Build history of the part. All positions in model axes, mm. Round coordinates to 2 decimals unless told otherwise and drop trailing zeros. Write each loop counter-clockwise with the first axis right and the second up, starting at its lowest first coordinate (ties: lowest second). Pieces come first, ordered by that corner, then holes. Notation, with made-up numbers: (89, 60.25) -> (97, 60.25) arc R26 ccw to (97, 96.25) -> close; hole circle Ø2 at (-17, 74.25). An arc over 180 degrees is marked (long way). Answer in a Markdown table with one row per item.
```python
from build123d import *

# Parameters (mm, degrees)
BOSS_EXTRUDE1_DEPTH        = 914.4
SKETCH2_R                  = 22.225
CUT_EXTRUDE1_DEPTH         = 917.272215283
F_1_2_0_5_DIAMETER_HOLE1_D = 12.7


with BuildPart() as part:
    # Sketch1 → Boss-Extrude1 (new body)
    with BuildSketch(Plane.XY):
        with BuildLine():
            Line((41.45, -19.05), (-41.45, -19.05))
            ThreePointArc((-41.45, -19.05), (-43.571320344, -18.171320344), (-44.45, -16.05))
            Line((-44.45, -16.05), (-44.45, 16.05))
            ThreePointArc((-44.45, 16.05), (-43.571320344, 18.171320344), (-41.45, 19.05))
            Line((-41.45, 19.05), (41.45, 19.05))
            ThreePointArc((41.45, 19.05), (43.571320344, 18.171320344), (44.45, 16.05))
            Line((44.45, 16.05), (44.45, -16.05))
            ThreePointArc((44.45, -16.05), (43.571320344, -18.171320344), (41.45, -19.05))
        make_face()
    extrude(amount=BOSS_EXTRUDE1_DEPTH)

    # Sketch2 → Cut-Extrude1 (cut, through all)
    with BuildSketch(Plane(origin=(0, 19.05, 0), x_dir=(1, 0, 0), z_dir=(0, 1, 0))):
        with Locations(Location((0, -304.8, 0), (0, 0, 180))):
            Circle(SKETCH2_R)
    extrude(amount=-CUT_EXTRUDE1_DEPTH, mode=Mode.SUBTRACT)

    # 1/2 (0.5) Diameter Hole1 (through all)
    with Locations(Plane(origin=(0, 19.05, 0), x_dir=(1, 0, 0), z_dir=(0, 1, 0))):
        with Locations((-25.4, -895.35), (25.4, -895.35), (-25.4, -19.05), (25.4, -19.05)):
            Hole(F_1_2_0_5_DIAMETER_HOLE1_D / 2)


solid = part.part
```
Q1. Saw through at C-C on y = 6. Write the cut outline in (x, z) (3 decimals).
A:
| item | result |
|---|---|
| outline | (-44.45, 0) -> (44.45, 0) -> (44.45, 914.4) -> (-44.45, 914.4) -> close; hole circle Ø12.7 at (-25.4, 19.05); hole circle Ø12.7 at (-25.4, 895.35); hole circle Ø44.45 at (0, 304.8); hole circle Ø12.7 at (25.4, 19.05); hole circle Ø12.7 at (25.4, 895.35) |
Q2. Saw through at B-B on z = 304.8. Write the cut outline in (x, y) (3 decimals), plus the area to 3 significant figures.
A:
| item | result |
|---|---|
| outline | (-44.45, -16.05) arc R3 ccw to (-41.45, -19.05) -> (-22.225, -19.05) -> (-22.225, 19.05) -> (-41.45, 19.05) arc R3 ccw to (-44.45, 16.05) -> close; (22.225, -19.05) -> (41.45, -19.05) arc R3 ccw to (44.45, -16.05) -> (44.45, 16.05) arc R3 ccw to (41.45, 19.05) -> (22.225, 19.05) -> close |
| area | 1,690 mm² |
Q3. Wall check: line 1 (Z direction, x = 24, y = -5.5); line 2 (Z direction, x = 25, y = -9); line 3 (X direction, y = -1, z = 895). Give the ranges that are in metal, low to high. Write a range as [from, to].
A:
| item | result |
|---|---|
| line 1 | [0, 12.86], [25.24, 889.16], [901.54, 914.4] |
| line 2 | [0, 12.71], [25.39, 889.01], [901.69, 914.4] |
| line 3 | [-44.45, -31.74], [-19.06, 19.06], [31.74, 44.45] |
Q4. Two-plate mould, pull along X, no slides. Class faces 1 (the flat face through (44.45, 0, 451)), 2 (the cylindrical face through (4.8, 0.3, 283.1)), 3 (the flat face through (-44.45, 0, 451)): released by +X, released by -X, zero draft, split by the parting line, or undercut.
A:
| item | result |
|---|---|
| face 1 | released by +X |
| face 2 | undercut |
| face 3 | released by -X |
Q5. Drop a flat-ended pin along its axis: P1, Ø10, axis at x = 33.5, y = -15, coming from the -Z side. Give the stop position or say it passes through.
A:
| item | result |
|---|---|
| P1 | z = 0 |
Q6. Saw through at A-A on x = 0. Write the cut outline in (y, z) (3 decimals).
A:
| item | result |
|---|---|
| outline | (-19.05, 0) -> (19.05, 0) -> (19.05, 282.575) -> (-19.05, 282.575) -> close; (-19.05, 327.025) -> (19.05, 327.025) -> (19.05, 914.4) -> (-19.05, 914.4) -> close |
